```python
from build123d import *
from OCP.BRepFilletAPI import BRepFilletAPI_MakeChamfer

# Parameters (mm, degrees)
SKETCH1_W           = 76.2
SKETCH1_H           = 76.2
BOSS_EXTRUDE1_DEPTH = 25.4
SKETCH2_W           = 57.15
SKETCH2_H           = 57.15
CUT_EXTRUDE1_DEPTH  = 19.05
BOSS_EXTRUDE2_DEPTH = 12.7
CHAMFER1_SIZE       = 2.54
CHAMFER1_SIZE2      = 1.27


with BuildPart() as part:
    # Sketch1 → Boss-Extrude1 (new body)
    with BuildSketch(Plane(origin=(0, 1478.617106037, 0), x_dir=(1, 0, 0), z_dir=(0, 1, 0))):
        with Locations((-492.049198231, -806.92955637)):
            Rectangle(SKETCH1_W, SKETCH1_H)
    extrude(amount=BOSS_EXTRUDE1_DEPTH)

    # Sketch2 → Cut-Extrude1 (cut)
    with BuildSketch(Plane(origin=(0, 1478.617106037, 0), x_dir=(-1, 0, 0), z_dir=(0, -1, 0))):
        with Locations((492.049198231, -806.92955637)):
            Rectangle(SKETCH2_W, SKETCH2_H)
    extrude(amount=-CUT_EXTRUDE1_DEPTH, mode=Mode.SUBTRACT)

    # Sketch3 → Boss-Extrude2 (add)
    with BuildSketch(Plane(origin=(0, 1478.617106037, 0), x_dir=(-1, 0, 0), z_dir=(0, -1, 0))):
        Polygon((530.149198231, -790.41955637), (527.482198231, -790.41955637), (527.482198231, -771.49655637), (508.559198231, -771.49655637), (508.559198231, -768.82955637), (530.149198231, -768.82955637), align=None)
        Polygon((530.149198231, -823.43955637), (527.482198231, -823.43955637), (527.482198231, -842.36255637), (508.559198231, -842.36255637), (508.559198231, -845.02955637), (530.149198231, -845.02955637), align=None)
        Polygon((475.539198231, -768.82955637), (475.539198231, -771.49655637), (456.616198231, -771.49655637), (456.616198231, -790.41955637), (453.949198231, -790.41955637), (453.949198231, -768.82955637), align=None)
        Polygon((475.539198231, -845.02955637), (475.539198231, -842.36255637), (456.616198231, -842.36255637), (456.616198231, -823.43955637), (453.949198231, -823.43955637), (453.949198231, -845.02955637), align=None)
    extrude(amount=BOSS_EXTRUDE2_DEPTH)

    # Chamfer1: one chamfer whose edges measure the first distance from different faces: ONE call of the kernel's chamfer builder (chamfer() names one face for all edges)
    chamfer1_edges_1 = [part.edges().sort_by_distance(p)[0] for p in [
        (-518.020698231, 1465.917106037, 771.49655637),
    ]]
    chamfer1_side_1 = [part.faces().sort_by_distance(p)[0] for p in [
        (-518.020698231, 1472.267106037, 771.49655637),
    ]]
    chamfer1_edges_2 = [part.edges().sort_by_distance(p)[0] for p in [
        (-527.482198231, 1465.917106037, 780.95805637),
    ]]
    chamfer1_side_2 = [part.faces().sort_by_distance(p)[0] for p in [
        (-527.482198231, 1472.267106037, 780.95805637),
    ]]
    chamfer1_edges_3 = [part.edges().sort_by_distance(p)[0] for p in [
        (-527.482198231, 1465.917106037, 832.90105637),
    ]]
    chamfer1_side_3 = [part.faces().sort_by_distance(p)[0] for p in [
        (-527.482198231, 1472.267106037, 832.90105637),
    ]]
    chamfer1_edges_4 = [part.edges().sort_by_distance(p)[0] for p in [
        (-518.020698231, 1465.917106037, 842.36255637),
    ]]
    chamfer1_side_4 = [part.faces().sort_by_distance(p)[0] for p in [
        (-518.020698231, 1472.267106037, 842.36255637),
    ]]
    chamfer1_edges_5 = [part.edges().sort_by_distance(p)[0] for p in [
        (-466.077698231, 1465.917106037, 771.49655637),
    ]]
    chamfer1_side_5 = [part.faces().sort_by_distance(p)[0] for p in [
        (-466.077698231, 1472.267106037, 771.49655637),
    ]]
    chamfer1_edges_6 = [part.edges().sort_by_distance(p)[0] for p in [
        (-456.616198231, 1465.917106037, 780.95805637),
    ]]
    chamfer1_side_6 = [part.faces().sort_by_distance(p)[0] for p in [
        (-456.616198231, 1472.267106037, 780.95805637),
    ]]
    chamfer1_edges_7 = [part.edges().sort_by_distance(p)[0] for p in [
        (-466.077698231, 1465.917106037, 842.36255637),
    ]]
    chamfer1_side_7 = [part.faces().sort_by_distance(p)[0] for p in [
        (-466.077698231, 1472.267106037, 842.36255637),
    ]]
    chamfer1_edges_8 = [part.edges().sort_by_distance(p)[0] for p in [
        (-456.616198231, 1465.917106037, 832.90105637),
    ]]
    chamfer1_side_8 = [part.faces().sort_by_distance(p)[0] for p in [
        (-456.616198231, 1472.267106037, 832.90105637),
    ]]
    chamfer1 = BRepFilletAPI_MakeChamfer(part.part.solid().wrapped)
    for e in chamfer1_edges_1:
        chamfer1.Add(CHAMFER1_SIZE, CHAMFER1_SIZE2, e.wrapped, chamfer1_side_1[0].wrapped)  # the first distance lies on this face
    for e in chamfer1_edges_2:
        chamfer1.Add(CHAMFER1_SIZE, CHAMFER1_SIZE2, e.wrapped, chamfer1_side_2[0].wrapped)  # the first distance lies on this face
    for e in chamfer1_edges_3:
        chamfer1.Add(CHAMFER1_SIZE, CHAMFER1_SIZE2, e.wrapped, chamfer1_side_3[0].wrapped)  # the first distance lies on this face
    for e in chamfer1_edges_4:
        chamfer1.Add(CHAMFER1_SIZE, CHAMFER1_SIZE2, e.wrapped, chamfer1_side_4[0].wrapped)  # the first distance lies on this face
    for e in chamfer1_edges_5:
        chamfer1.Add(CHAMFER1_SIZE, CHAMFER1_SIZE2, e.wrapped, chamfer1_side_5[0].wrapped)  # the first distance lies on this face
    for e in chamfer1_edges_6:
        chamfer1.Add(CHAMFER1_SIZE, CHAMFER1_SIZE2, e.wrapped, chamfer1_side_6[0].wrapped)  # the first distance lies on this face
    for e in chamfer1_edges_7:
        chamfer1.Add(CHAMFER1_SIZE, CHAMFER1_SIZE2, e.wrapped, chamfer1_side_7[0].wrapped)  # the first distance lies on this face
    for e in chamfer1_edges_8:
        chamfer1.Add(CHAMFER1_SIZE, CHAMFER1_SIZE2, e.wrapped, chamfer1_side_8[0].wrapped)  # the first distance lies on this face
    add(Compound.cast(chamfer1.Shape()), mode=Mode.REPLACE)


solid = part.part
```
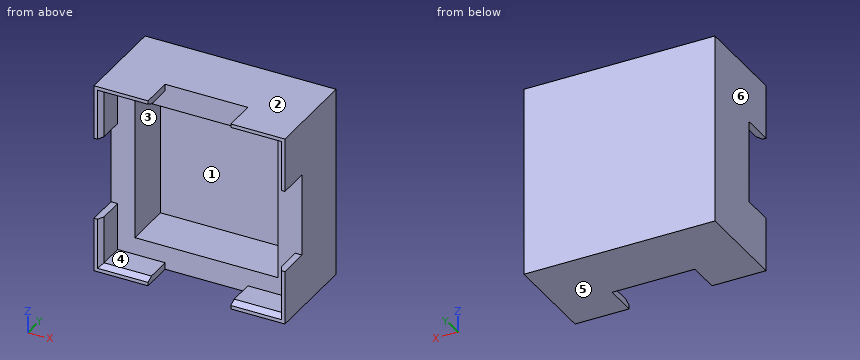
CAD build for the part. Positions are in the model's coordinates, mm. Face numbers are marked on the shaded views. A direction names the side the tool comes from. Coordinates: 2 decimals unless noted, no trailing zeros. Order: outer loops, then holes, each group sorted by start corner. A loop starts at its lowest first (then second) coordinate and runs counter-clockwise, first axis right, second up.
(1) Saw through at D-D, the plane z = 825. Write the cut outline in (x, y), and give its area (3 significant figures).
Solution:
outline: (-530.15, 1465.92) - (-528.75, 1465.92) - (-527.48, 1468.46) - (-527.48, 1478.62) - (-520.62, 1478.62) - (-520.62, 1497.67) - (-463.47, 1497.67) - (-463.47, 1478.62) - (-456.62, 1478.62) - (-456.62, 1468.46) - (-455.35, 1465.92) - (-453.95, 1465.92) - (-453.95, 1504.02) - (-530.15, 1504.02) - close
area: 911 mm2
(2) Drill centre lines: L1, parallel to X at y = 1489, z = 796; L2, parallel to X at y = 1469, z = 826; L3, parallel to Z at x = -490, y = 1496.5. Where is each one in solid material? Low to high.
Solution:
L1: x = -530.15 to -520.62, -463.47 to -453.95
L2: x = -530.15 to -527.48, -456.62 to -453.95
L3: z = 768.83 to 778.35, 835.5 to 845.03
(3) Which spindle directions (+Z, -Z, +X, -X, +Y, -Y) get a long thin tool onto all of the face, cutting with end or side? Do the marked faces 1 and 2. Say none if no direction does.
Solution:
face 1: -Y
face 2: +Z, +X, -X, +Y, -Y
(4) Mould opens along Z. For the marked faces 3, 4, 5 and 6 say: released by +Z, released by -Z, zero draft, split by the parting line, or undercut.
Solution:
face 3: undercut
face 4: undercut
face 5: released by -Z
face 6: zero draft
(5) Saw through at B-B, the plane y = 1477.5. Write the cut outline in (x, z).
Solution:
outline: (-530.15, 768.83) - (-508.56, 768.83) - (-508.56, 771.5) - (-527.48, 771.5) - (-527.48, 790.42) - (-530.15, 790.42) - close; (-530.15, 823.44) - (-527.48, 823.44) - (-527.48, 842.36) - (-508.56, 842.36) - (-508.56, 845.03) - (-530.15, 845.03) - close; (-475.54, 768.83) - (-453.95, 768.83) - (-453.95, 790.42) - (-456.62, 790.42) - (-456.62, 771.5) - (-475.54, 771.5) - close; (-475.54, 842.36) - (-456.62, 842.36) - (-456.62, 823.44) - (-453.95, 823.44) - (-453.95, 845.03) - (-475.54, 845.03) - close
(6) Saw through at C-C, the plane x = -512.5. Write the cut outline in (y, z), and give its area (3 significant figures).
Solution:
outline: (1465.92, 768.83) - (1504.02, 768.83) - (1504.02, 845.03) - (1465.92, 845.03) - (1465.92, 843.63) - (1468.46, 842.36) - (1478.62, 842.36) - (1478.62, 835.5) - (1497.67, 835.5) - (1497.67, 778.35) - (1478.62, 778.35) - (1478.62, 771.5) - (1468.46, 771.5) - (1465.92, 770.23) - close
area: 911 mm2
(7) Pin check, flat tip, straight feed: pin 1 Ø1.5 at (x, z) = (-476, 833.5) entering from -Y. Stop position of the tip, or through.
Solution:
pin 1: stops at y = 1497.67
(8) Saw through at A-A, the plane y = 1490. Write the cut outline in (x, z).
Solution:
outline: (-530.15, 768.83) - (-453.95, 768.83) - (-453.95, 845.03) - (-530.15, 845.03) - close; hole (-520.62, 778.35) - (-463.47, 778.35) - (-463.47, 835.5) - (-520.62, 835.5) - close
